from build123d import *

# Parameters (mm, degrees)
CYLINDER001_R           = 3
CYLINDER001_DEPTH       = 4.06
CYLINDER003_R           = 0.89
CYLINDER003_DEPTH       = 2.79
CYLINDER002_R           = 2.29
CYLINDER002_DEPTH       = 2.79
BOX_W                   = 10
BOX_H                   = 1.4
BOX_DEPTH               = 10
CYLINDER004_R           = 1
CYLINDER004_DEPTH       = 10
PAD_DEPTH               = 6
CYLINDER005_R           = 0.64
CYLINDER005_DEPTH       = 5
CYLINDER005_PITCH_ANGLE = 90
CYLINDER006_R           = 0.64
CYLINDER006_DEPTH       = 5
CYLINDER006_PITCH_ANGLE = 90
CYLINDER007_R           = 0.64
CYLINDER007_DEPTH       = 5
CYLINDER007_PITCH_ANGLE = 90
CYLINDER_R              = 6
CYLINDER_DEPTH          = 4.06


with BuildPart() as cylinder001:
    # Cylinder001 → Cylinder001 (new body)
    with BuildSketch(Plane(origin=(-0.57, 0, 6.22), x_dir=(1, 0, 0), z_dir=(0, 0, 1))):
        Circle(CYLINDER001_R)
    extrude(amount=CYLINDER001_DEPTH)


with BuildPart() as cylinder003:
    # Cylinder003 → Cylinder003 (new body)
    with BuildSketch(Plane(origin=(5.43, 0, 10.28), x_dir=(1, 0, 0), z_dir=(0, 0, 1))):
        Circle(CYLINDER003_R)
    extrude(amount=CYLINDER003_DEPTH)


with BuildPart() as cut:
    # Cylinder002 → Cylinder002 (new body)
    with BuildSketch(Plane(origin=(5.43, 0, 10.28), x_dir=(1, 0, 0), z_dir=(0, 0, 1))):
        Circle(CYLINDER002_R)
    extrude(amount=CYLINDER002_DEPTH)

    # Cut: cut Cylinder003
    add(cylinder003.part, mode=Mode.SUBTRACT)


with BuildPart() as box:
    # Box → Box (new body)
    with BuildSketch(Plane(origin=(14, -0.7, -3), x_dir=(1, 0, 0), z_dir=(0, 0, 1))):
        with Locations((5, 0.7)):
            Rectangle(BOX_W, BOX_H)
    extrude(amount=BOX_DEPTH)


with BuildPart() as part_mirroring001:
    # Part__Mirroring001: instance of Box
    add(box.part.mirror(Plane(origin=(0, 0, 0), x_dir=(0, -1, 0), z_dir=(1, 0, 0))))


with BuildPart() as cylinder004:
    # Cylinder004 → Cylinder004 (new body)
    with BuildSketch(Plane(origin=(14, 0, -3), x_dir=(1, 0, 0), z_dir=(0, 0, 1))):
        Circle(CYLINDER004_R)
    extrude(amount=CYLINDER004_DEPTH)


with BuildPart() as fusion:
    # Part__Mirroring: instance of Cylinder004
    add(cylinder004.part.mirror(Plane(origin=(0, 0, 0), x_dir=(0, -1, 0), z_dir=(1, 0, 0))))

    # Fusion: union Part__Mirroring001, Cylinder004, Box
    add(part_mirroring001.part)
    add(cylinder004.part)
    add(box.part)


with BuildPart() as cut001:
    # Sketch → Pad (new body, symmetric)
    with BuildSketch(Plane.XZ):
        Polygon((16.256, 1.143), (16.256, -1.143), (11.43, -1.143), (11.43, -16.891), (-11.43, -16.891), (-11.43, -1.143), (-16.256, -1.143), (-16.256, 1.143), (-11.43, 1.143), (-11.43, 6.223), (11.43, 6.223), (11.43, 1.143), align=None)
    extrude(amount=PAD_DEPTH, both=True)

    # Cut001: cut Fusion
    add(fusion.part, mode=Mode.SUBTRACT)


with BuildPart() as cylinder005:
    # Cylinder005 → Cylinder005 (new body)
    with BuildSketch(Plane.XY):
        Circle(CYLINDER005_R)
    extrude(amount=CYLINDER005_DEPTH)


with BuildPart() as cylinder005_1:
    # Cylinder005 pitch: moved
    add(cylinder005.part.rotate(Axis((0, 0, 0), (0, 1, 0)), CYLINDER005_PITCH_ANGLE))


with BuildPart() as cylinder005_2:
    # Cylinder005 placement: moved
    add(cylinder005_1.part.moved(Location((11.43, 0, -12))))


with BuildPart() as cylinder006:
    # Cylinder006 → Cylinder006 (new body)
    with BuildSketch(Plane.XY):
        Circle(CYLINDER006_R)
    extrude(amount=CYLINDER006_DEPTH)


with BuildPart() as cylinder006_1:
    # Cylinder006 pitch: moved
    add(cylinder006.part.rotate(Axis((0, 0, 0), (0, 1, 0)), CYLINDER006_PITCH_ANGLE))


with BuildPart() as cylinder006_2:
    # Cylinder006 placement: moved
    add(cylinder006_1.part.moved(Location((11.43, -1.28, -12))))


with BuildPart() as cylinder007:
    # Cylinder007 → Cylinder007 (new body)
    with BuildSketch(Plane.XY):
        Circle(CYLINDER007_R)
    extrude(amount=CYLINDER007_DEPTH)


with BuildPart() as cylinder007_1:
    # Cylinder007 pitch: moved
    add(cylinder007.part.rotate(Axis((0, 0, 0), (0, 1, 0)), CYLINDER007_PITCH_ANGLE))


with BuildPart() as cylinder007_2:
    # Cylinder007 placement: moved
    add(cylinder007_1.part.moved(Location((11.43, 1.28, -12))))


with BuildPart() as obj1:
    # Cylinder → Cylinder (new body)
    with BuildSketch(Plane(origin=(5.43, 0, 6.22), x_dir=(1, 0, 0), z_dir=(0, 0, 1))):
        Circle(CYLINDER_R)
    extrude(amount=CYLINDER_DEPTH)

    # Fusion001: union Cylinder001, Cut, Cut001, Cylinder005, Cylinder006, Cylinder007
    add(cylinder001.part)
    add(cut.part)
    add(cut001.part)
    add(cylinder005_2.part)
    add(cylinder006_2.part)
    add(cylinder007_2.part)


solid = obj1.part
Geometry: final body of the model. Coordinates: model frame, mm. A direction names the side the tool comes from. Round coordinates to 2 decimals unless told otherwise and drop trailing zeros. Loops run counter-clockwise (first coordinate to the right, second up) from the corner with the lowest first, then second, coordinate; pieces in that order, holes last.
Q1. Pin query (flat end, axial travel): P1, Ø6.5, axis at x = 8.5, y = 1.5, coming from the +Z side; P2, Ø2, axis at x = 13, y = -2.5, coming from the -Z side; P3, Ø1.4, axis at x = -13, y = 1, coming from the +Z side; P4, Ø1, axis at y = -2.5, z = 8, coming from the +X side. Return the tip coordinate at first contact, or that it passes through.
Q2. Pull-direction query (Y, two-part tool) for faces 4 (the cylindrical face through (13.9, -0.01, -12.64)), 5 (the flat face through (-12.8, -0.1, 1.143)), 6 (the cylindrical face through (11.426, -0.221, 8.223)); classes: released by +Y, released by -Y, zero draft, split by the parting line, or undercut.
Q3. Material intervals for L1, parallel to Y at x = -14, z = -0.25; L2, parallel to Y at x = 5.43, z = 11.65; L3, parallel to X at y = -3, z = -4, sorted ascending.
Q4. Section D-D on x = -10.5. Return loops of the section in (y, z), plus the area to 3 significant figures.
Q5. Access query for faces 1 (the flat face through (10, 5, 6.223)), 2 (the flat face through (-11.43, 0, -9)), 3 (the flat face through (-15, 0.7, 0)). Directions: +Z, -Z, +X, -X, +Y, -Y. A direction counts if a zero-diameter tool reaches every point of the face in a straight line with its end or side. Return the directions, or none.
Q6. Section C-C on z = -14.5. Return loops of the section in (x, y), plus the area to 3 significant figures.
Q7. Section B-B on x = -0.57. Return loops of the section in (y, z).
Evaluation:
1. P1: stops at z = 13.07
1. P2: stops at z = -12.6
1. P3: stops at z = 1.14
1. P4: stops at x = 11.09
2. face 4: undercut
2. face 5: zero draft
2. face 6: split by the parting line
3. L1: y = -6 to -1, 1 to 6
3. L2: y = -2.29 to -0.89, 0.89 to 2.29
3. L3: x = -11.43 to 11.43
4. outline: (-6, -16.89) - (6, -16.89) - (6, 6.22) - (-6, 6.22) - close
4. area: 277 mm2
5. face 1: +Z, +X, +Y
5. face 2: -Z, -X, +Y, -Y
5. face 3: +Z, -Z, -X
6. outline: (-11.43, -6) - (11.43, -6) - (11.43, 6) - (-11.43, 6) - close
6. area: 274 mm2
7. outline: (-6, -16.89) - (6, -16.89) - (6, 6.22) - (3, 6.22) - (3, 10.28) - (-3, 10.28) - (-3, 6.22) - (-6, 6.22) - close
